from build123d import *

# Parameters (mm, degrees)
BOSS_EXTRUDE1_DEPTH    = 50.8
F_12_28_TAPPED_HOLE1_D = 4.6228
SKETCH6_W              = 50.8
SKETCH6_H              = 27.94
BOSS_EXTRUDE2_DEPTH    = 11.43


with BuildPart() as part:
    # Sketch2 → Boss-Extrude1 (new body)
    with BuildSketch(Plane(origin=(0, 0, 0), x_dir=(1, 0, 0), z_dir=(0, 1, 0))):
        Polygon((0, 0), (0, 50.8), (3.175, 50.8), (3.175, 3.175), (31.75, 3.175), (31.75, 0), align=None)
    extrude(amount=BOSS_EXTRUDE1_DEPTH)

    # #12-28 Tapped Hole1 (through all)
    with Locations(Plane(origin=(0, 0, -3.175), x_dir=(-1, 0, 0), z_dir=(0, 0, -1))):
        with Locations((-17.4625, 25.4)):
            Hole(F_12_28_TAPPED_HOLE1_D / 2)

    # Sketch6 → Boss-Extrude2 (add)
    with BuildSketch(Plane.ZY):
        with Locations((-25.4, 25.4)):
            Rectangle(SKETCH6_W, SKETCH6_H)
    extrude(amount=BOSS_EXTRUDE2_DEPTH)


solid = part.part
Check sheet for the modelled part. Datum: model origin and axes. Units: mm. A direction names the side the tool comes from. Round coordinates to 2 decimals unless told otherwise and drop trailing zeros. Loops run counter-clockwise (first coordinate to the right, second up) from the corner with the lowest first, then second, coordinate; pieces in that order, holes last.
1. Sectioned sample at C-C on y = 13.5. Record the boundary of the cut face in (x, z) (3 decimals).
2. Scan lines: probe 1 along X at (y, z) = (9, -49) (3 decimals); probe 2 along X at (y, z) = (20, -31) (3 decimals); probe 3 along Z at (x, y) = (5, 35.5) (3 decimals). Record each from-to range of solid material in increasing order.
3. Sectioned sample at A-A on y = 25.4. Record the boundary of the cut face in (x, z) (3 decimals), and give its area (3 significant figures).
4. Mould release check, pull along X, two halves, no side actions. Record for faces 6 (the flat face through (31.75, 25, -2)), 7 (the flat face through (10, 25, 0)), 8 (the cylindrical face through (17.16, 27.69, -1.57)): released by +X, released by -X, zero draft, split by the parting line, or undercut.
5. Sectioned sample at D-D on x = 28. Record the boundary of the cut face in (y, z) (3 decimals).
6. Set-up check for faces 1 (the flat face through (3.175, 25, -27)), 2 (the flat face through (-3, 25, -50.8)), 3 (the flat face through (-6, 11.43, -26)), 4 (the flat face through (0, 45, -25)), 5 (the flat face through (3, 0, -16)): record each of +Z, -Z, +X, -X, +Y, -Y from which the full face is reachable in a straight line by a thin tool's end or side.
7. Gauge pin test, flat ends, axial feed: pin 1 Ø12.5 at (x, z) = (-5, -32.5) entering from -Y; pin 2 Ø8 at (x, z) = (-5, -37.5) entering from +Y; pin 3 Ø3.5 at (y, z) = (8.5, -25.5) entering from -X; pin 4 Ø3 at (x, y) = (19.5, 12) entering from -Z (3 decimals). Record the tip position at first contact, or that the pin passes through.
8. Sectioned sample at B-B on z = -48. Record the boundary of the cut face in (x, y) (3 decimals), and give its area (3 significant figures).
Recorded:
1. outline: (-11.43, -50.8) - (3.175, -50.8) - (3.175, -3.175) - (31.75, -3.175) - (31.75, 0) - (-11.43, 0) - close
2. probe 1: x = 0 to 3.175
2. probe 2: x = -11.43 to 3.175
2. probe 3: z = -3.175 to 0
3. outline: (-11.43, -50.8) - (3.175, -50.8) - (3.175, -3.175) - (15.151, -3.175) - (15.151, 0) - (-11.43, 0) - close; (19.774, -3.175) - (31.75, -3.175) - (31.75, 0) - (19.774, 0) - close
3. area: 818 mm2
4. face 6: released by +X
4. face 7: zero draft
4. face 8: undercut
5. outline: (0, -3.175) - (50.8, -3.175) - (50.8, 0) - (0, 0) - close
6. face 1: -Z, +X, +Y, -Y
6. face 2: -Z, +X, -X, +Y, -Y
6. face 3: +Z, -Z, -X, -Y
6. face 4: +Z, -Z, -X, +Y
6. face 5: +Z, -Z, +X, -X, -Y
7. pin 1: stops at y = 0
7. pin 2: stops at y = 39.37
7. pin 3: stops at x = 0
7. pin 4: stops at z = -3.175
8. outline: (-11.43, 11.43) - (0, 11.43) - (0, 0) - (3.175, 0) - (3.175, 50.8) - (0, 50.8) - (0, 39.37) - (-11.43, 39.37) - close
8. area: 481 mm2
